Geometry: final body of the model. Coordinates: model frame, mm. A direction names the side the tool comes from. Round coordinates to 2 decimals unless told otherwise and drop trailing zeros. Write each loop counter-clockwise with the first axis right and the second up, starting at its lowest first coordinate (ties: lowest second). Pieces come first, ordered by that corner, then holes. Notation, with made-up numbers: (56, 65.5) -> (104, 65.5) arc R14 cw to (104, 90.5) -> close; hole circle Ø10 at (89.25, -34). An arc over 180 degrees is marked (long way). Use one line per item in the form item = value. Start each with the question number.
1. Draft query along Z for faces 3 (the face through (-1.5, -0.27, 9.93)), 4 (the face through (0, 0, 16)), 5 (the face through (0, 0, 0)). Return one class per face: pulls with the +Z half, pulls with the -Z half, needs draft (parallel to the pull), parting line crosses it, or undercut.
2. Cut plane A-A, the plane x = 0. Return the cut outline in (y, z), plus the area to 3 significant figures.
3. Reachability of faces 1 (the face through (0, -3, 8)), 2 (the face through (-1.2, 2.384, 11.4)) from +Z, -Z, +X, -X, +Y, -Y: full face, straight path, thin tool, end or side. Return the list, or none.
4. Cut plane C-C, the plane z = 10. Return the cut outline in (x, y).
5. Pin query (flat end, axial travel): pin 1 Ø1.1 at (x, z) = (-1, 9.5) entering from +Y; pin 2 Ø1.8 at (x, z) = (0, 10) entering from -Y; pin 3 Ø2 at (y, z) = (-2, 7.5) entering from -X. Return the tip coordinate at first contact, or that it passes through.
6. Line query: L1, parallel to Z at x = 0, y = 0.5; L2, parallel to X at y = -0.05, z = 10; L3, parallel to X at y = 1.15, z = 10. Output: solid intervals per line, ascending.
7. Cut plane B-B, the plane y = -0.25. Return the cut outline in (x, z).
8. Cut plane D-D, the plane z = 3.75. Return the cut outline in (x, y).
Autodesk Inventor part; units mm, degrees
ref_plane "YZ Plane" through (0, 0, 0) normal (1, 0, 0) x (0, 1, 0)
ref_plane "XZ Plane" through (0, 0, 0) normal (0, 1, 0) x (-1, 0, 0)
ref_plane "XY Plane" through (0, 0, 0) normal (0, 0, 1) x (1, 0, 0)
sketch "Sketch1" plane through (0, 0, 0) normal (0, 0, 1) x (1, 0, 0)
  circle A0 centre (0, 0) radius 3
  circle A1 centre (0, 0) radius 5
  dimension "d0" = 10
  dimension "d1" = 6
extrude "Extrusion1" add sketch "Sketch1" along normal blind 16 contours A0
sketch "Sketch2" plane through (0, 0, 16) normal (0, 0, 1) x (1, 0, 0)
  circle A0 centre (0, 0) radius 3
  line L0 (-1.8209, 2.3842) -> (1.8209, 2.3842)
  line L1 (-3, 0) -> (3, 0)
extrude "Extrusion2" cut sketch "Sketch2" against normal blind 12 contours L0 A0
sketch "Sketch3" plane through (-1.8209, 2.3842, 16) normal (0, 1, 0) x (1, 0, 0)
  circle A0 centre (1.8209, 6) radius 1.5
  line L0 (3.6417, 0) -> (0, 0)
  point P0 (1.8209, 16)
  dimension "d6" = 6
  dimension "d7" = 3
extrude "Extrusion3" cut sketch "Sketch3" against normal up to surface
thread "Thread1"
properties part number "motor shaft" material "Steel, Mild"
Outcome:
q1.face_3 = undercut
q1.face_4 = pulls with the +Z half
q1.face_5 = pulls with the -Z half
q2.outline = (-3, 0) -> (3, 0) -> (3, 4) -> (2.38, 4) -> (2.38, 8.5) -> (-3, 8.5) -> close; (-3, 11.5) -> (2.38, 11.5) -> (2.38, 16) -> (-3, 16) -> close
q2.area = 72.5 mm^2
q3.face_1 = +Z, -Z
q3.face_2 = +Z, +X, -X, +Y
q4.outline = (-1.82, 2.38) arc R3 ccw to (-1.5, -2.6) -> (-1.5, 2.38) -> close; (1.5, -2.6) arc R3 ccw to (1.82, 2.38) -> (1.5, 2.38) -> close
q5.pin_1 = 2.38
q5.pin_2 = through
q5.pin_3 = -2.83
q6.L1 = 0 to 8.5, 11.5 to 16
q6.L2 = -3 to -1.5, 1.5 to 3
q6.L3 = -2.77 to -1.5, 1.5 to 2.77
q7.outline = (-2.99, 0) -> (2.99, 0) -> (2.99, 16) -> (-2.99, 16) -> close; hole circle Ø3 at (0, 10)
q8.outline = circle Ø6 at (0, 0)
